```python
from build123d import *

# Parameters (mm, degrees)
SKETCH1_W               = 41.275
SKETCH1_H               = 88.9
BOSS_EXTRUDE1_DEPTH     = 5.9944
SKETCH1_5_W             = 8.89
SKETCH1_5_H             = 88.9
BOSS_EXTRUDE2_DEPTH     = 12.3444
SKETCH3_R               = 2.2225
CUT_EXTRUDE1_DEPTH      = 1
CUT_EXTRUDE1_DEPTH_BACK = 13.3444
SKETCH4_R               = 3.683
CUT_EXTRUDE2_DEPTH      = 4.064
SKETCH5_W               = 2.54
SKETCH5_H               = 88.9
CUT_EXTRUDE3_DEPTH      = 7.35
CUT_EXTRUDE3_DEPTH_BACK = 6.9944
BOSS_EXTRUDE3_DEPTH     = 88.9
CUT_EXTRUDE4_DEPTH      = 88.9


with BuildPart() as part:
    # Sketch1 → Boss-Extrude1 (new body)
    with BuildSketch(Plane(origin=(0, 0, 0), x_dir=(1, 0, 0), z_dir=(0, 1, 0))):
        with Locations((20.6375, 44.45)):
            Rectangle(SKETCH1_W, SKETCH1_H)
    extrude(amount=BOSS_EXTRUDE1_DEPTH)

    # Sketch1<5> → Boss-Extrude2 (add)
    with BuildSketch(Plane(origin=(0, 0, 0), x_dir=(1, 0, 0), z_dir=(0, 1, 0))):
        with Locations((45.72, 44.45)):
            Rectangle(SKETCH1_5_W, SKETCH1_5_H)
    extrude(amount=BOSS_EXTRUDE2_DEPTH)

    # Sketch3 → Cut-Extrude1 (cut, two sides)
    with BuildSketch(Plane(origin=(0, 12.3444, 0), x_dir=(1, 0, 0), z_dir=(0, 1, 0))) as cut_extrude1_sk:
        with Locations((45.72, 82.55)):
            Circle(SKETCH3_R)
        with Locations((45.72, 6.35)):
            Circle(SKETCH3_R)
    extrude(amount=CUT_EXTRUDE1_DEPTH, mode=Mode.SUBTRACT)
    extrude(cut_extrude1_sk.sketch, amount=-CUT_EXTRUDE1_DEPTH_BACK, mode=Mode.SUBTRACT)

    # Sketch4 → Cut-Extrude2 (cut)
    with BuildSketch(Plane.XZ):
        with Locations((45.72, -6.35)):
            Circle(SKETCH4_R)
        with Locations((45.72, -82.55)):
            Circle(SKETCH4_R)
    extrude(amount=-CUT_EXTRUDE2_DEPTH, mode=Mode.SUBTRACT)

    # Sketch5 → Cut-Extrude3 (cut, two sides)
    with BuildSketch(Plane(origin=(0, 5.9944, 0), x_dir=(1, 0, 0), z_dir=(0, 1, 0))) as cut_extrude3_sk:
        with Locations((1.27, 44.45)):
            Rectangle(SKETCH5_W, SKETCH5_H)
    extrude(amount=CUT_EXTRUDE3_DEPTH, mode=Mode.SUBTRACT)
    extrude(cut_extrude3_sk.sketch, amount=-CUT_EXTRUDE3_DEPTH_BACK, mode=Mode.SUBTRACT)

    # Sketch6 → Boss-Extrude3 (add)
    with BuildSketch(Plane.XY):
        Polygon((2.54, 6.2484), (2.54, 5.9944), (21.9075, 5.9944), align=None)
    extrude(amount=-BOSS_EXTRUDE3_DEPTH)

    # Sketch6<3> → Cut-Extrude4 (cut)
    with BuildSketch(Plane.XY):
        Polygon((41.275, 5.9944), (21.9075, 5.9944), (41.275, 5.7404), align=None)
    extrude(amount=-CUT_EXTRUDE4_DEPTH, mode=Mode.SUBTRACT)


solid = part.part
```
Geometry check sheet. Reference: the model listing, model coordinates, mm. A direction names the side the tool comes from. Coordinates: 2 decimals unless noted, no trailing zeros. Order: outer loops, then holes, each group sorted by start corner. A loop starts at its lowest first (then second) coordinate and runs counter-clockwise, first axis right, second up.
Item 1: Section check C-C (y = 1). Enter the section's corners in (x, z) (3 decimals), plus the area to 3 significant figures.
Item 2: Section check B-B (z = -6.35). Enter the section's corners in (x, y) (1 decimal).
Item 3: Depth check by flat-ended pin: pin 1 (4 mm diameter, centred on x = 45.72, z = -82.55, fed in from -Y); pin 2 (4 mm diameter, centred on x = 39, z = -56, fed in from +Y); pin 3 (3.5 mm diameter, centred on x = 44.5, z = -84, fed in from -Y); pin 4 (6 mm diameter, centred on x = 17.5, z = -76, fed in from +Y). Enter the tip coordinate at first touch or a pass-through.
Item 4: Section check A-A (x = 45.72). Enter the section's corners in (y, z).
Item 5: Section check D-D (z = -73.5). Enter the section's corners in (x, y) (3 decimals), plus the area to 3 significant figures.
Item 6: Scan lines: line 1 along Z through (x, y) = (45.72, 6.5); line 2 along Z through (x, y) = (45.72, 0.9); line 3 along X through (y, z) = (5.5, -6.35) (1 decimal). Record each from-to range of solid material in increasing order.
Item 7: Tool access check on faces 1 (the cylindrical face through (43.5, 8.3, -6.4)), 2 (the flat face through (46, 4.064, -9)). Record the directions out of +Z, -Z, +X, -X, +Y, -Y that give a thin tool (end or side, any length) a straight path to the whole face; none if there is none.
Item 8: Mould release check, pull along Z, two halves, no side actions. Record for faces 3 (the flat face through (31, 4, 0)), 4 (the cylindrical face through (45.24, 8.26, -80.38)), 5 (the flat face through (50.165, 6, -44)), 6 (the flat face through (48.1, 4.064, -82.5)): released by +Z, released by -Z, zero draft, split by the parting line, or undercut.
Check sheet entries:
1. outline: (2.54, -88.9) - (50.165, -88.9) - (50.165, 0) - (2.54, 0) - close; hole circle Ø7.366 at (45.72, -82.55); hole circle Ø7.366 at (45.72, -6.35)
1. area: 4,150 mm2
2. outline: (2.5, 0) - (42, 0) - (42, 4.1) - (43.5, 4.1) - (43.5, 12.3) - (41.3, 12.3) - (41.3, 5.7) - (2.5, 6.2) - close; (47.9, 4.1) - (49.4, 4.1) - (49.4, 0) - (50.2, 0) - (50.2, 12.3) - (47.9, 12.3) - close
3. pin 1: passes through
3. pin 2: stops at y = 5.8
3. pin 3: stops at y = 4.06
3. pin 4: stops at y = 6.09
4. outline: (0, -88.9) - (12.34, -88.9) - (12.34, -84.77) - (4.06, -84.77) - (4.06, -86.23) - (0, -86.23) - close; (0, -78.87) - (4.06, -78.87) - (4.06, -80.33) - (12.34, -80.33) - (12.34, -8.57) - (4.06, -8.57) - (4.06, -10.03) - (0, -10.03) - close; (0, -2.67) - (4.06, -2.67) - (4.06, -4.13) - (12.34, -4.13) - (12.34, 0) - (0, 0) - close
5. outline: (2.54, 0) - (50.165, 0) - (50.165, 12.344) - (41.275, 12.344) - (41.275, 5.74) - (2.54, 6.248) - close
5. area: 342 mm2
6. line 1: z = -88.9 to -84.77, -80.33 to -8.57, -4.13 to 0
6. line 2: z = -88.9 to -86.23, -78.87 to -10.03, -2.67 to 0
6. line 3: x = 2.5 to 43.5, 47.9 to 50.2
7. face 1: +Y, -Y
7. face 2: -Y
8. face 3: released by +Z
8. face 4: undercut
8. face 5: zero draft
8. face 6: undercut
